Can you work these out from the drawing? Everything is in mm from the part's minimum corner. A direction names the side the tool comes from. Coordinates: 2 decimals unless noted, no trailing zeros. Order: outer loops, then holes, each group sorted by start corner. A loop starts at its lowest first (then second) coordinate and runs counter-clockwise, first axis right, second up. Notation, with made-up numbers: M -23.5,-11.75 L 4.5,-11.75 A18 cw 4.5,18.25 Z; hole C 26,-23.5 d9. An arc over 180 degrees is marked long. Answer as a JSON object with one key per item and string values.
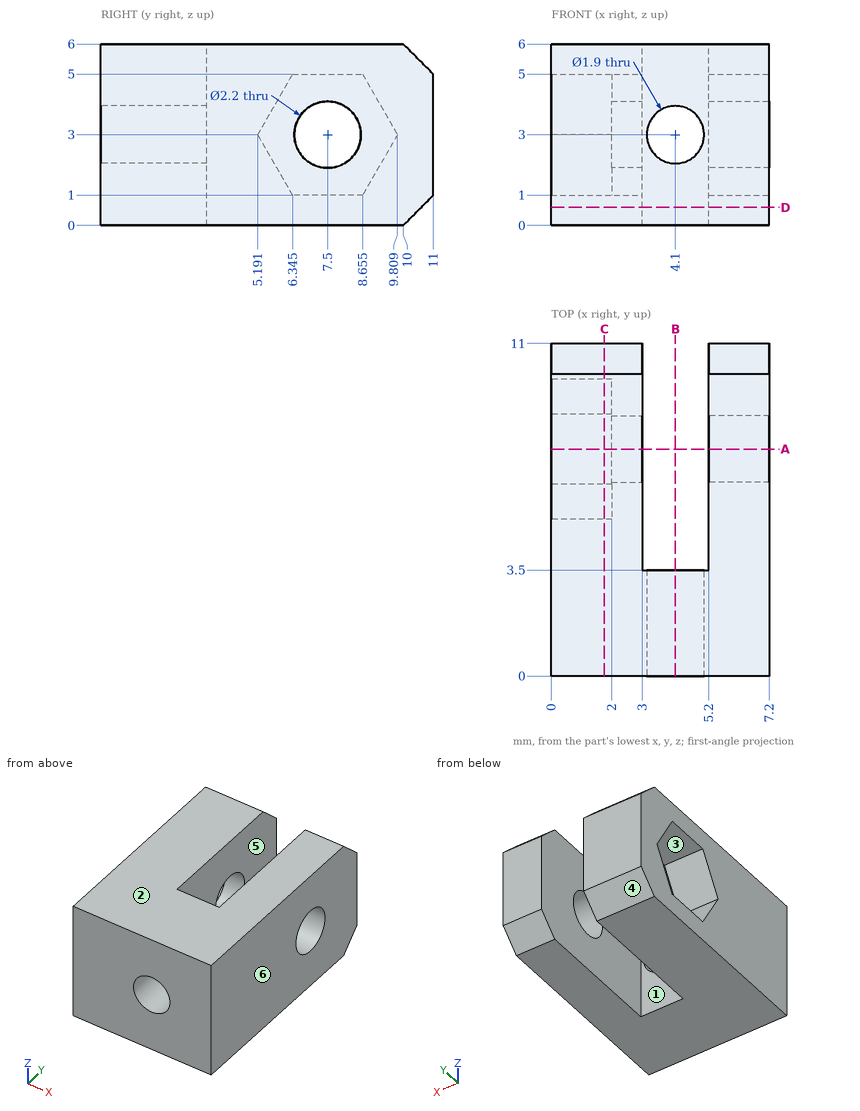
Item 1: I want a section at B-B, the plane x = 4.1. Write out the boundary of the cut face in (y, z).
Answers follow:
{"outline": "M 0,0 L 3.5,0 L 3.5,2.05 L 0,2.05 Z; M 0,3.95 L 3.5,3.95 L 3.5,6 L 0,6 Z"}
Item 2: I want a section at C-C, the plane x = 1.75. Write out the boundary of the cut face in (y, z) (1 decimal).
Answers follow:
{"outline": "M 0,0 L 10,0 L 11,1 L 11,5 L 10,6 L 0,6 Z; hole M 5.2,3 L 6.3,1 L 8.7,1 L 9.8,3 L 8.7,5 L 6.3,5 Z"}
Item 3: If we mould it in two halves opening along X, with no side actions, what happens to the marked faces 4, 5 and 6? For each: pulls with the +X half, pulls with the -X half, needs draft (parallel to the pull), parting line crosses it, or undercut.
Answers follow:
{"face 4": "needs draft", "face 5": "undercut", "face 6": "pulls with the +X half"}
Item 4: I'm going to push flat-ended pins straight in: pin 1 (1.1 mm diameter, centred on x = 4, z = 3.5, fed in from +Y); pin 2 (3.5 mm diameter, centred on y = 7.5, z = 3, fed in from -X). Where does each tip first touch, or does it pass through?
Answers follow:
{"pin 1": "stops at y = 3.5", "pin 2": "stops at x = 2"}
Item 5: Please list where these lines run through material, in increasing order: line 1 (Y direction, x = 5.75, z = 3); line 2 (X direction, y = 5, z = 2.25); line 3 (Y direction, x = 5, z = 4.9).
Answers follow:
{"line 1": "y = 0 to 6.4, 8.6 to 11", "line 2": "x = 0 to 3, 5.2 to 7.2", "line 3": "y = 0 to 3.5"}
Item 6: I want a section at A-A, the plane y = 7.5. Write out the boundary of the cut face in (x, z).
Answers follow:
{"outline": "M 0,0 L 3,0 L 3,1.9 L 2,1.9 L 2,1 L 0,1 Z; M 0,5 L 2,5 L 2,4.1 L 3,4.1 L 3,6 L 0,6 Z; M 5.2,0 L 7.2,0 L 7.2,1.9 L 5.2,1.9 Z; M 5.2,4.1 L 7.2,4.1 L 7.2,6 L 5.2,6 Z"}
Item 7: Which directions (+Z, -Z, +X, -X, +Y, -Y) give clear straight access to the entire face, cutting with the end or side of a thin tool? Please do the marked faces 1, 2 and 3.
Answers follow:
{"face 1": "+Z, -Z, +Y", "face 2": "+Z, +X, -X, +Y, -Y", "face 3": "-X"}
Item 8: I want a section at D-D, the plane z = 0.6. Write out the boundary of the cut face in (x, y).
Answers follow:
{"outline": "M 0,0 L 7.2,0 L 7.2,10.6 L 5.2,10.6 L 5.2,3.5 L 3,3.5 L 3,10.6 L 0,10.6 Z"}
